Check sheet for the modelled part. Datum: model origin and axes. Units: mm. Give positions to 0.01 mm unless a question says otherwise; leave off trailing zeros. Order: outer loops, then holes, each group sorted by start corner. A loop starts at its lowest first (then second) coordinate and runs counter-clockwise, first axis right, second up.
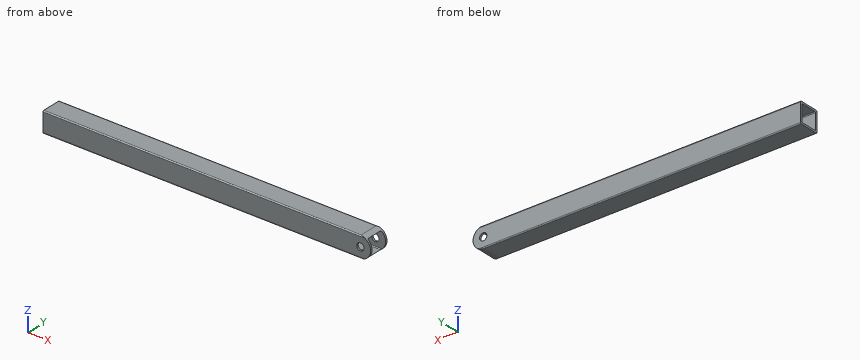
```python
from build123d import *

# Parameters (mm, degrees)
BOSS_EXTRUDE1_DEPTH      = 152.4
BOSS_EXTRUDE1_DEPTH_BACK = 152.4
CUT_EXTRUDE1_DEPTH       = 154.881084364
SKETCH6_R                = 3.3782
CUT_EXTRUDE2_DEPTH       = 154.881084481


with BuildPart() as part:
    # Sketch4 → Boss-Extrude1 (new, two sides: drawn at the far end of the back side and taken through both)
    with BuildSketch(Plane(origin=(0, 0, 0), x_dir=(0, 0, -1), z_dir=(1, 0, 0)).offset(-BOSS_EXTRUDE1_DEPTH_BACK)):
        with BuildLine():
            Line((9.525, -8.5725), (9.525, 8.5725))
            ThreePointArc((9.525, 8.5725), (9.246019209, 9.246019209), (8.5725, 9.525))
            Line((8.5725, 9.525), (-8.5725, 9.525))
            ThreePointArc((-8.5725, 9.525), (-9.246019209, 9.246019209), (-9.525, 8.5725))
            Line((-9.525, 8.5725), (-9.525, -8.5725))
            ThreePointArc((-9.525, -8.5725), (-9.246019209, -9.246019209), (-8.5725, -9.525))
            Line((-8.5725, -9.525), (8.5725, -9.525))
            ThreePointArc((8.5725, -9.525), (9.246019209, -9.246019209), (9.525, -8.5725))
        make_face()
        with BuildLine():
            Line((7.874, 7.0866), (7.874, -7.0866))
            ThreePointArc((7.874, -7.0866), (7.64337588, -7.64337588), (7.0866, -7.874))
            Line((7.0866, -7.874), (-7.0866, -7.874))
            ThreePointArc((-7.0866, -7.874), (-7.64337588, -7.64337588), (-7.874, -7.0866))
            Line((-7.874, -7.0866), (-7.874, 7.0866))
            ThreePointArc((-7.874, 7.0866), (-7.64337588, 7.64337588), (-7.0866, 7.874))
            Line((-7.0866, 7.874), (7.0866, 7.874))
            ThreePointArc((7.0866, 7.874), (7.64337588, 7.64337588), (7.874, 7.0866))
        make_face(mode=Mode.SUBTRACT)
    extrude(amount=BOSS_EXTRUDE1_DEPTH + BOSS_EXTRUDE1_DEPTH_BACK)

    # Sketch5 → Cut-Extrude1 (cut, through all)
    with BuildSketch(Plane.XZ.offset(9.525)):
        with BuildLine():
            Line((152.4, -9.525), (142.875, -9.525))
            ThreePointArc((142.875, -9.525), (152.4, 0), (142.875, 9.525))
            Line((142.875, 9.525), (152.4, 9.525))
            Line((152.4, 9.525), (157.48, 9.525))
            Line((157.48, 9.525), (157.48, -9.525))
            Line((157.48, -9.525), (152.4, -9.525))
        make_face()
    extrude(amount=-CUT_EXTRUDE1_DEPTH, mode=Mode.SUBTRACT)

    # Sketch6 → Cut-Extrude2 (cut, through all)
    with BuildSketch(Plane(origin=(0, 9.525, 0), x_dir=(1, 0, 0), z_dir=(0, 1, 0))):
        with Locations(Location((142.875, 0, 0), (0, 0, 270))):
            Circle(SKETCH6_R)
    extrude(amount=-CUT_EXTRUDE2_DEPTH, mode=Mode.SUBTRACT)


solid = part.part
```
(1) Sectioned sample at A-A (y = -3.5). Enter the section's corners in (x, z) (3 decimals).
(2) Sectioned sample at C-C (z = 0). Enter the section's corners in (x, y) (3 decimals).
(3) Thickness scan on L1, parallel to Y at x = -114, z = 5 (3 decimals); L2, parallel to X at y = 8.65, z = 0. Record the ranges inside material, lowest first.
(4) Sectioned sample at B-B (x = 73). Enter the section's corners in (y, z) (1 decimal).
(5) Go/stop test with a flat-tipped pin: P1, Ø8, axis at y = -7, z = 6.5, coming from the +X side. Record where the tip stops, or that it passes through.
Values follow:
1. outline: (-152.4, -9.525) - (142.875, -9.525) arc R9.525 ccw to (148.235, -7.874) - (-152.4, -7.874) - close; (-152.4, 7.874) - (148.235, 7.874) arc R9.525 ccw to (142.875, 9.525) - (-152.4, 9.525) - close
2. outline: (-152.4, -9.525) - (139.497, -9.525) - (139.497, -7.874) - (-152.4, -7.874) - close; (-152.4, 7.874) - (139.497, 7.874) - (139.497, 9.525) - (-152.4, 9.525) - close; (146.253, -9.525) - (152.4, -9.525) - (152.4, -7.874) - (146.253, -7.874) - close; (146.253, 7.874) - (152.4, 7.874) - (152.4, 9.525) - (146.253, 9.525) - close
3. L1: y = -9.525 to -7.874, 7.874 to 9.525
3. L2: x = -152.4 to 139.5, 146.25 to 152.4
4. outline: (-9.5, -8.6) arc R1 ccw to (-8.6, -9.5) - (8.6, -9.5) arc R1 ccw to (9.5, -8.6) - (9.5, 8.6) arc R1 ccw to (8.6, 9.5) - (-8.6, 9.5) arc R1 ccw to (-9.5, 8.6) - close; hole (-7.9, -7.1) arc R0.8 ccw to (-7.1, -7.9) - (7.1, -7.9) arc R0.8 ccw to (7.9, -7.1) - (7.9, 7.1) arc R0.8 ccw to (7.1, 7.9) - (-7.1, 7.9) arc R0.8 ccw to (-7.9, 7.1) - close
5. P1: stops at x = 152.04
